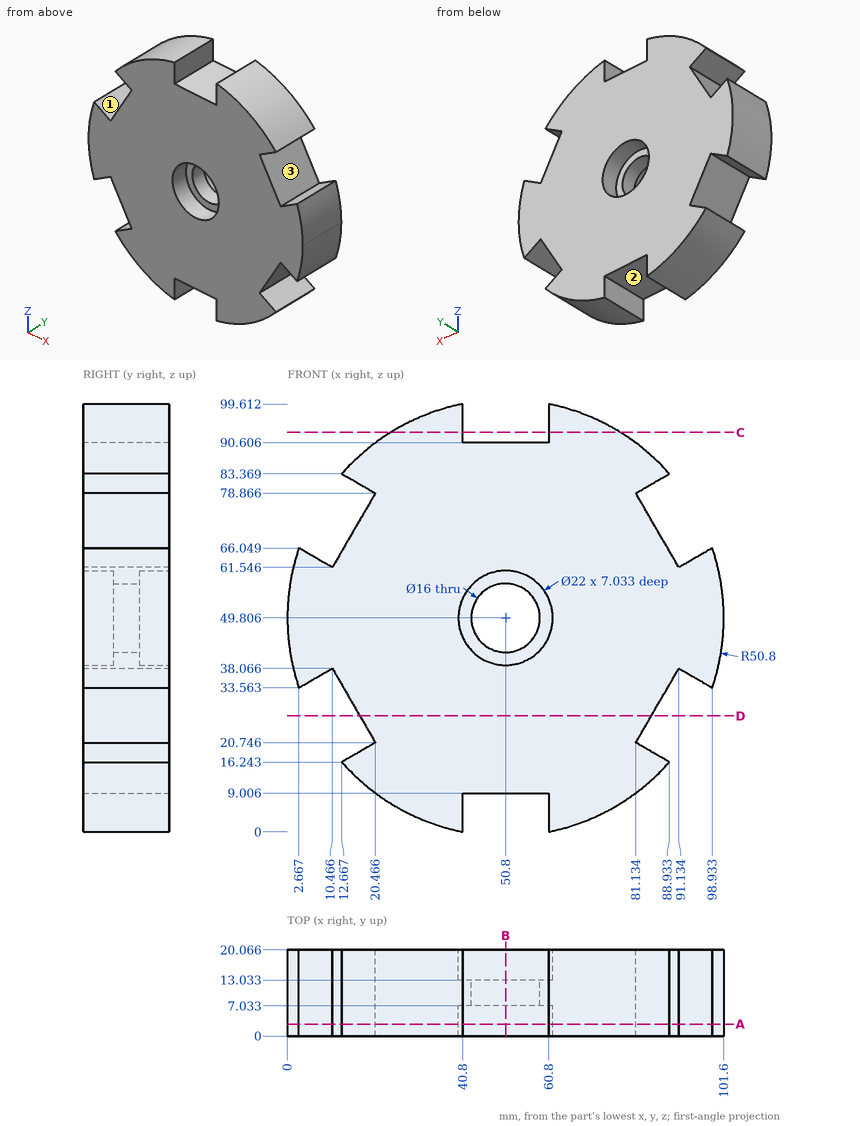
Part print with two shaded views. Sizes in mm from the minimum x, y, z corner. A direction names the side the tool comes from. Round coordinates to 2 decimals unless told otherwise and drop trailing zeros. Order: outer loops, then holes, each group sorted by start corner. A loop starts at its lowest first (then second) coordinate and runs counter-clockwise, first axis right, second up. Notation, with made-up numbers: M -14,70.5 L 23,70.5 A11 cw 23,77.5 Z; hole C 56.5,32 d11. An arc over 180 degrees is marked long. Use CSV: the item, a comma, the result in double quotes.
Item 1: Saw through at B-B (x = 50.8). List the corners of the cut face in (y, z).
Worked answers:
outline,"M 0,9.01 L 20.07,9.01 L 20.07,38.81 L 13.03,38.81 L 13.03,41.81 L 7.03,41.81 L 7.03,38.81 L 0,38.81 Z; M 0,60.81 L 7.03,60.81 L 7.03,57.81 L 13.03,57.81 L 13.03,60.81 L 20.07,60.81 L 20.07,90.61 L 0,90.61 Z"
Item 2: Saw through at C-C (z = 93). List the corners of the cut face in (x, y), plus the area to 3 significant figures.
Worked answers:
outline,"M 24.06,0 L 40.8,0 L 40.8,20.07 L 24.06,20.07 Z; M 60.8,0 L 77.54,0 L 77.54,20.07 L 60.8,20.07 Z"
area,"672 mm²"
Item 3: Saw through at A-A (y = 2.75). List the corners of the cut face in (x, z), plus the area to 3 significant figures.
Worked answers:
outline,"M 2.67,33.56 L 10.47,38.07 L 20.47,20.75 L 12.67,16.24 A50.8 ccw 40.8,0 L 40.8,9.01 L 60.8,9.01 L 60.8,0 A50.8 ccw 88.93,16.24 L 81.13,20.75 L 91.13,38.07 L 98.93,33.56 A50.8 ccw 101.6,49.81 A50.8 ccw 98.93,66.05 L 91.13,61.55 L 81.13,78.87 L 88.93,83.37 A50.8 ccw 60.8,99.61 L 60.8,90.61 L 40.8,90.61 L 40.8,99.61 A50.8 ccw 12.67,83.37 L 20.47,78.87 L 10.47,61.55 L 2.67,66.05 A50.8 ccw Z; hole C 50.8,49.81 d22"
area,"6,570 mm²"
Item 4: Probe probe 1 along Z at (x, y) = (50.8, 8.8); probe 2 along Z at (x, y) = (50.8, 5.25); probe 3 along X at (y, z) = (4.5, 37). List the from-to ranges inside material, lowest first.
Worked answers:
probe 1,"9.01 to 41.81, 57.81 to 90.61"
probe 2,"9.01 to 38.81, 60.81 to 90.61"
probe 3,"1.64 to 8.62, 11.08 to 90.52, 92.98 to 99.96"
Item 5: Saw through at D-D (z = 27). List the corners of the cut face in (x, y) (1 decimal), plus the area to 3 significant figures.
Worked answers:
outline,"M 16.9,0 L 84.7,0 L 84.7,20.1 L 16.9,20.1 Z"
area,"1,360 mm²"
Item 6: Which spindle directions (+Z, -Z, +X, -X, +Y, -Y) get a long thin tool onto all of the face, cutting with end or side? Do the marked faces 1, 2 and 3. Say none if no direction does.
Worked answers:
face 1,"+Z, +Y, -Y"
face 2,"-Z, +Y, -Y"
face 3,"+Y, -Y"
Item 7: Pin check, flat tips, straight feed: pin 1 (17.5 mm diameter, centred on x = 50.8, z = 49.81, fed in from +Y); pin 2 (6 mm diameter, centred on x = 47.5, y = 8.5, fed in from -Z); pin 3 (4.5 mm diameter, centred on y = 14.5, z = 94, fed in from -X); pin 4 (24 mm diameter, centred on x = 48, z = 51, fed in from +Y). Stop position of each tip, or through.
Worked answers:
pin 1,"y = 13.03"
pin 2,"z = 9.01"
pin 3,"x = 22.14"
pin 4,"y = 20.07"
